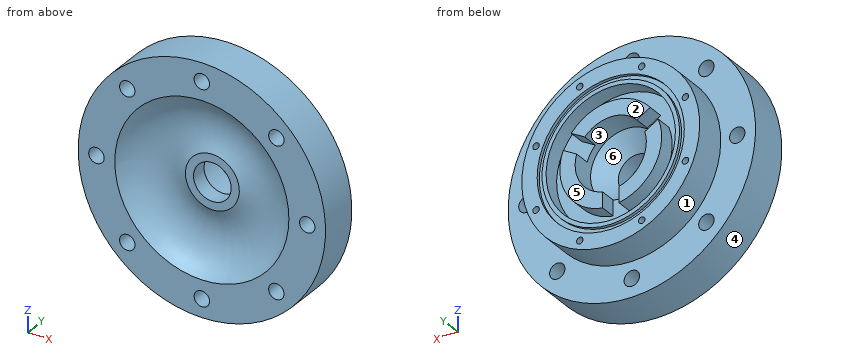
```python
from build123d import *

# Parameters (mm, degrees)
SKETCH4_R          = 4.7625
CUT_EXTRUDE2_DEPTH = 114.707959264
CIRPATTERN1_COUNT  = 8
SKETCH6_R          = 40
SKETCH6_R_2        = 31.5
CUT_EXTRUDE3_DEPTH = 10
SKETCH7_W          = 10
SKETCH7_H          = 10.050043706
CUT_EXTRUDE4_DEPTH = 10
CIRPATTERN2_COUNT  = 3
SKETCH9_R          = 2
CUT_EXTRUDE5_DEPTH = 10
CIRPATTERN3_COUNT  = 8
SKETCH10_R         = 45.5
SKETCH10_R_2       = 42.5
CUT_EXTRUDE6_DEPTH = 2


with BuildPart() as part:
    # Sketch3 → Revolve1 (revolve)
    with BuildSketch(Plane(origin=(0, 0, 0), x_dir=(0, 0, -1), z_dir=(1, 0, 0))):
        with BuildLine():
            Line((76.5, 15), (55, 15))
            Line((55, 15), (55, 35))
            Line((55, 35), (22.025, 35))
            Line((22.025, 35), (22.025, 20.36))
            Line((22.025, 20.36), (11.665, 10))
            Line((11.665, 10), (11.665, 0))
            Line((11.665, 0), (16.665, 0))
            ThreePointArc((16.665, 0), (37.471852779, 3.234070807), (53.85, -10))
            Line((53.85, -10), (76.5, -10))
            Line((76.5, -10), (76.5, 15))
        make_face()
    revolve(axis=Axis((0, 0, 0), (0, 1, 0)))

    # Sketch4 → Cut-Extrude2 (cut, symmetric)
    with BuildSketch(Plane(origin=(0, 0, 0), x_dir=(1, 0, 0), z_dir=(0, 1, 0))):
        with Locations(Location((-65.2, 0, 0), (0, 0, 270))):
            Circle(SKETCH4_R)
    cut_extrude2 = extrude(amount=CUT_EXTRUDE2_DEPTH, both=True, mode=Mode.SUBTRACT)

    # CirPattern1: Cut-Extrude2 ×8 about axis
    cirpattern1_axis = Axis((0, 0, 0), (0, 1, 0))
    for i in range(1, CIRPATTERN1_COUNT):
        add(cut_extrude2.rotate(cirpattern1_axis, i * 360 / CIRPATTERN1_COUNT), mode=Mode.SUBTRACT)

    # Sketch6 → Cut-Extrude3 (cut)
    with BuildSketch(Plane(origin=(0, 35, 0), x_dir=(1, 0, 0), z_dir=(0, 1, 0))):
        with Locations(Location((0, 0, 0), (0, 0, 270))):
            Circle(SKETCH6_R)
        with Locations(Location((0, 0, 0), (0, 0, 270))):
            Circle(SKETCH6_R_2, mode=Mode.SUBTRACT)
    extrude(amount=-CUT_EXTRUDE3_DEPTH, mode=Mode.SUBTRACT)

    # Sketch7 → Cut-Extrude4 (cut)
    with BuildSketch(Plane(origin=(0, 35, 0), x_dir=(1, 0, 0), z_dir=(0, 1, 0))):
        with Locations((0, 26.474978147)):
            Rectangle(SKETCH7_W, SKETCH7_H)
    cut_extrude4 = extrude(amount=-CUT_EXTRUDE4_DEPTH, mode=Mode.SUBTRACT)

    # CirPattern2: Cut-Extrude4 ×3 about axis
    cirpattern2_axis = Axis((0, 0, 0), (0, 1, 0))
    for i in range(1, CIRPATTERN2_COUNT):
        add(cut_extrude4.rotate(cirpattern2_axis, i * 360 / CIRPATTERN2_COUNT), mode=Mode.SUBTRACT)

    # Sketch9 → Cut-Extrude5 (cut)
    with BuildSketch(Plane(origin=(0, 35, 0), x_dir=(1, 0, 0), z_dir=(0, 1, 0))):
        with Locations(Location((46.193976626, 19.134171618, 0), (0, 0, 270))):
            Circle(SKETCH9_R)
    cut_extrude5 = extrude(amount=-CUT_EXTRUDE5_DEPTH, mode=Mode.SUBTRACT)

    # CirPattern3: Cut-Extrude5 ×8 about axis
    cirpattern3_axis = Axis((0, 0, 0), (0, 1, 0))
    for i in range(1, CIRPATTERN3_COUNT):
        add(cut_extrude5.rotate(cirpattern3_axis, i * 360 / CIRPATTERN3_COUNT), mode=Mode.SUBTRACT)

    # Sketch10 → Cut-Extrude6 (cut)
    with BuildSketch(Plane(origin=(0, 35, 0), x_dir=(1, 0, 0), z_dir=(0, 1, 0))):
        with Locations(Location((0, 0, 0), (0, 0, 270))):
            Circle(SKETCH10_R)
        with Locations(Location((0, 0, 0), (0, 0, 270))):
            Circle(SKETCH10_R_2, mode=Mode.SUBTRACT)
    extrude(amount=-CUT_EXTRUDE6_DEPTH, mode=Mode.SUBTRACT)


solid = part.part
```
Verification items for the finished model (mm, model axes). Face numbers are marked on the shaded views. A direction names the side the tool comes from. Give positions to 0.01 mm unless a question says otherwise; leave off trailing zeros. Order: outer loops, then holes, each group sorted by start corner. A loop starts at its lowest first (then second) coordinate and runs counter-clockwise, first axis right, second up. Notation, with made-up numbers: M 62.5,-22 L 93.5,-22 A20 ccw 93.5,-17 Z; hole C 20.5,17 d10. An arc over 180 degrees is marked long. Answer in a Markdown table with one row per item. Add a question column.
Item 1: Section check B-B, the plane x = 65.2. Enter the section's corners in (y, z), and give its area (3 significant figures).
Item 2: Section check A-A, the plane z = -65.2. Enter the section's corners in (x, y).
Item 3: Scan lines: probe 1 along X at (y, z) = (5, 0) (1 decimal); probe 2 along X at (y, z) = (30.75, 0) (3 decimals); probe 3 along Z at (x, y) = (8.5, 26). Record each from-to range of solid material in increasing order. Write a range as from..to.
Item 4: Gauge pin test, flat ends, axial feed: pin 1 (15 mm diameter, centred on x = 0, z = -65.2, fed in from -Y); pin 2 (12 mm diameter, centred on x = 41.5, y = 30, fed in from +Z); pin 3 (4.5 mm diameter, centred on x = -19.13, z = 46.19, fed in from -Y); pin 4 (4 mm diameter, centred on y = 22.5, z = 48.5, fed in from +X). Record the tip position at first contact, or that the pin passes through.
Item 5: Tool access check on the marked faces 1 and 2. Record the directions out of +Z, -Z, +X, -X, +Y, -Y that give a thin tool (end or side, any length) a straight path to the whole face; none if there is none.
Item 6: Section check C-C, the plane x = 0. State how many separate pieces and enclosed holes the cut face has, and give its area (3 significant figures).
Item 7: Mould release check, pull along Z, two halves, no side actions. Record for the marked faces 3, 4, 5 and 6: released by +Z, released by -Z, zero draft, split by the parting line, or undercut.
Filled sheet:
| question | item | result |
|---|---|---|
| 1 | outline | M -10,-40.02 L 15,-40.02 L 15,-4.76 L -10,-4.76 Z; M -10,4.76 L 15,4.76 L 15,40.02 L -10,40.02 Z |
| 1 | area | 1,760 mm^2 |
| 2 | outline | M -40.02,-10 L -4.76,-10 L -4.76,15 L -40.02,15 Z; M 4.76,-10 L 40.02,-10 L 40.02,15 L 4.76,15 Z |
| 3 | probe 1 | x = -76.5..-70, -60.4..-11.7, 11.7..60.4, 70..76.5 |
| 3 | probe 2 | x = -55..-40, -31.5..-22.025, 22.025..31.5, 40..55 |
| 3 | probe 3 | z = -54.34..-39.09, -30.33..-20.32, 20.32..30.33, 39.09..54.34 |
| 4 | pin 1 | stops at y = -10 |
| 4 | pin 2 | stops at z = 42.01 |
| 4 | pin 3 | stops at y = -7.29 |
| 4 | pin 4 | stops at x = 29.37 |
| 5 | face 1 | +Y |
| 5 | face 2 | +Z, -Z, +X, -X, +Y |
| 6 | separate pieces | 4 |
| 6 | enclosed holes | 0 |
| 6 | area | 2,890 mm^2 |
| 7 | face 3 | undercut |
| 7 | face 4 | split by the parting line |
| 7 | face 5 | zero draft |
| 7 | face 6 | undercut |
